```python
from build123d import *

# Parameters (mm, degrees)
F0_W     = 406.4
F0_H     = 254
F0_R     = 25.4
F0_W_2   = 76.2
F0_H_2   = 152.4
F0_W_3   = 25.4
F0_R_2   = 9.525
F1_DEPTH = 6.35
F3_DEPTH = 254.001
F5_DEPTH = 254.001


with BuildPart() as f1:
    # F0 (on Top) → F1 (new body)
    with BuildSketch(Plane.XY):
        with Locations((203.2, 127)):
            Rectangle(F0_W, F0_H)
        with Locations((279.4, 88.9)):
            Circle(F0_R, mode=Mode.SUBTRACT)
        with Locations((114.3, 127)):
            Rectangle(F0_W_2, F0_H_2, mode=Mode.SUBTRACT)
        with Locations((190.5, 127)):
            Rectangle(F0_W_3, F0_H_2, mode=Mode.SUBTRACT)
        with Locations((279.4, 165.1)):
            Circle(F0_R, mode=Mode.SUBTRACT)
        with Locations((317.5, 127)):
            Circle(F0_R_2, mode=Mode.SUBTRACT)
    extrude(amount=F1_DEPTH)

    # F2 (on face) → F3 (cut, through all)
    with BuildSketch(Plane.XZ):
        Polygon((2.3112109876, 0), (0, 6.35), (0, 0), align=None)
    extrude(amount=-F3_DEPTH, mode=Mode.SUBTRACT)

    # F4 (on face) → F5 (cut, through all)
    with BuildSketch(Plane.XZ):
        Polygon((400.05, 6.35), (402.3612109876, 0), (406.4, 0), (406.4, 6.35), align=None)
        Polygon((396.6623240103, 15.657563286), (400.05, 6.35), (406.4, 6.35), (406.4, 0), (417.733579874, 0), (417.733579874, 15.657563286), align=None)
    extrude(amount=-F5_DEPTH, mode=Mode.SUBTRACT)


solid = f1.part
```
Geometry check sheet. Reference: the model listing, model coordinates, mm. Coordinates: 2 decimals unless noted, no trailing zeros. Write each loop counter-clockwise with the first axis right and the second up, starting at its lowest first coordinate (ties: lowest second). Pieces come first, ordered by that corner, then holes. Notation, with made-up numbers: (2, 84.5) -> (61, 84.5) arc R21 ccw to (61, 100.5) -> close; hole circle Ø11 at (41, -37). An arc over 180 degrees is marked (long way). Use CSV: the item, a comma, the result in double quotes. Start each with the question number.
Item 1: Depth check by flat-ended pin: pin 1 Ø2 at (x, y) = (77, 128) entering from -Z; pin 2 Ø3 at (y, z) = (137.5, 3.5) entering from -X. Enter the tip coordinate at first touch or a pass-through.
Item 2: Mould release check, pull along X, two halves, no side actions. Record for faces 1 (the cylindrical face through (303.627, 172.729, 3.131)), 2 (the flat face through (244, 129, 0)): released by +X, released by -X, zero draft, split by the parting line, or undercut.
Item 3: Thickness scan on line 1 (Y direction, x = 279.4, z = 5.25); line 2 (Y direction, x = 135.5, z = 4.25); line 3 (Y direction, x = 260.5, z = 3). Record the ranges inside material, lowest first.
Item 4: Cross-section at A-A, the plane x = 135.5. Record the cut outline in (y, z).
Item 5: Cross-section at D-D, the plane z = 3.75. Record the cut outline in (x, y) (3 decimals).
Item 6: Cross-section at B-B, the plane y = 127. Record the cut outline in (x, z) (3 decimals), plus the area to 3 significant figures.
Item 7: Cross-section at C-C, the plane x = 279.4. Record the cut outline in (y, z), plus the area to 3 significant figures.
Answers:
1,pin 1,"z = 0"
1,pin 2,"x = 0.49"
2,face 1,"undercut"
2,face 2,"zero draft"
3,line 1,"0 to 63.5, 114.3 to 139.7, 190.5 to 254"
3,line 2,"0 to 50.8, 203.2 to 254"
3,line 3,"0 to 71.93, 105.87 to 148.13, 182.07 to 254"
4,outline,"(0, 0) -> (50.8, 0) -> (50.8, 6.35) -> (0, 6.35) -> close; (203.2, 0) -> (254, 0) -> (254, 6.35) -> (203.2, 6.35) -> close"
5,outline,"(0.946, 0) -> (400.996, 0) -> (400.996, 254) -> (0.946, 254) -> close; hole (76.2, 50.8) -> (152.4, 50.8) -> (152.4, 203.2) -> (76.2, 203.2) -> close; hole (177.8, 50.8) -> (203.2, 50.8) -> (203.2, 203.2) -> (177.8, 203.2) -> close; hole circle Ø50.8 at (279.4, 88.9); hole circle Ø50.8 at (279.4, 165.1); hole circle Ø19.05 at (317.5, 127)"
6,outline,"(0, 6.35) -> (2.311, 0) -> (76.2, 0) -> (76.2, 6.35) -> close; (152.4, 0) -> (177.8, 0) -> (177.8, 6.35) -> (152.4, 6.35) -> close; (203.2, 0) -> (307.975, 0) -> (307.975, 6.35) -> (203.2, 6.35) -> close; (327.025, 0) -> (402.361, 0) -> (400.05, 6.35) -> (327.025, 6.35) -> close"
6,area,"1,770 mm^2"
7,outline,"(0, 0) -> (63.5, 0) -> (63.5, 6.35) -> (0, 6.35) -> close; (114.3, 0) -> (139.7, 0) -> (139.7, 6.35) -> (114.3, 6.35) -> close; (190.5, 0) -> (254, 0) -> (254, 6.35) -> (190.5, 6.35) -> close"
7,area,"968 mm^2"
